Job drawing, mm, ordinate dimensions from the low corner. One solid piece. Coordinates: 2 decimals unless noted, no trailing zeros. Loops run counter-clockwise (first coordinate to the right, second up) from the corner with the lowest first, then second, coordinate; pieces in that order, holes last. Notation, with made-up numbers: (-20, 14.5) -> (22, 14.5) arc R12 cw to (22, 35.5) -> close; hole circle Ø3 at (41, 78). An arc over 180 degrees is marked (long way). Use one line per item in the form item = value. Start each with the question number.
(1) Drill centre lines: L1, parallel to Y at x = 2.5, z = 0.9; L2, parallel to X at y = 38.5, z = 1.4; L3, parallel to Y at x = 17.25, z = 1.85. Where is each one in solid material? Low to high. Write a range as [from, to].
(2) Band-saw the part on B-B on x = 2.5. Give the cut face in (y, z), then the cut area to 3 significant figures.
(3) Band-saw the part on C-C on y = 38.5. Give the cut face in (x, z), then the cut area to 3 significant figures.
(4) Band-saw the part on A-A on y = 2.5. Give the cut face in (x, z).
(5) Band-saw the part on D-D on z = 0.7. Give the cut face in (x, y).
(6) Pin check, flat tip, straight feed: P1, Ø2, axis at x = 26.5, y = 38.5, coming from the -Z side. Stop position of the tip, or through.
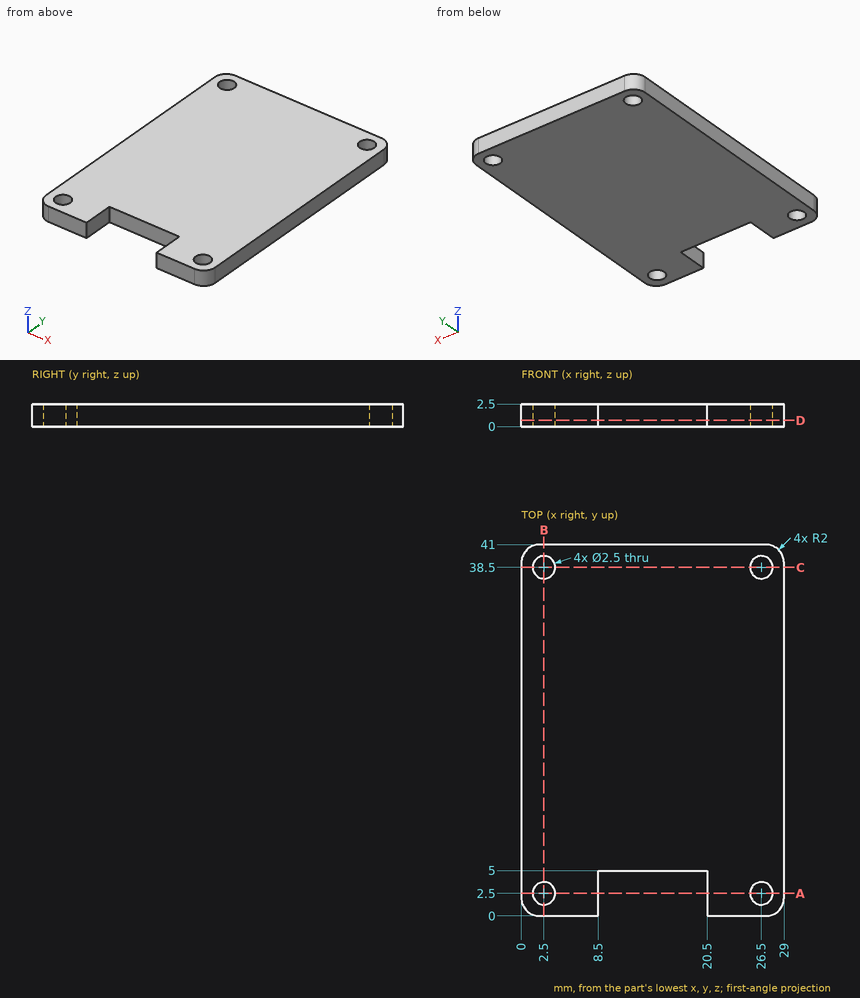
A:
q1.L1 = [0, 1.25], [3.75, 37.25], [39.75, 41]
q1.L2 = [0, 1.25], [3.75, 25.25], [27.75, 29]
q1.L3 = [5, 41]
q2.outline = (0, 0) -> (1.25, 0) -> (1.25, 2.5) -> (0, 2.5) -> close; (3.75, 0) -> (37.25, 0) -> (37.25, 2.5) -> (3.75, 2.5) -> close; (39.75, 0) -> (41, 0) -> (41, 2.5) -> (39.75, 2.5) -> close
q2.area = 90.0 mm²
q3.outline = (0, 0) -> (1.25, 0) -> (1.25, 2.5) -> (0, 2.5) -> close; (3.75, 0) -> (25.25, 0) -> (25.25, 2.5) -> (3.75, 2.5) -> close; (27.75, 0) -> (29, 0) -> (29, 2.5) -> (27.75, 2.5) -> close
q3.area = 60.0 mm²
q4.outline = (0, 0) -> (1.25, 0) -> (1.25, 2.5) -> (0, 2.5) -> close; (3.75, 0) -> (8.5, 0) -> (8.5, 2.5) -> (3.75, 2.5) -> close; (20.5, 0) -> (25.25, 0) -> (25.25, 2.5) -> (20.5, 2.5) -> close; (27.75, 0) -> (29, 0) -> (29, 2.5) -> (27.75, 2.5) -> close
q5.outline = (0, 2) arc R2 ccw to (2, 0) -> (8.5, 0) -> (8.5, 5) -> (20.5, 5) -> (20.5, 0) -> (27, 0) arc R2 ccw to (29, 2) -> (29, 39) arc R2 ccw to (27, 41) -> (2, 41) arc R2 ccw to (0, 39) -> close; hole circle Ø2.5 at (2.5, 2.5); hole circle Ø2.5 at (2.5, 38.5); hole circle Ø2.5 at (26.5, 2.5); hole circle Ø2.5 at (26.5, 38.5)
q6.P1 = through
